Verification items for the finished model (mm, model axes). A direction names the side the tool comes from. Give positions to 0.01 mm unless a question says otherwise; leave off trailing zeros. Write each loop counter-clockwise with the first axis right and the second up, starting at its lowest first coordinate (ties: lowest second). Pieces come first, ordered by that corner, then holes.
from build123d import *

# Parameters (mm, degrees)
SKETCH2_R               = 15.5
SKETCH2_R_2             = 14
BOSS_EXTRUDE1_DEPTH     = 20
SKETCH3_OUTSIDE_W       = 42.638
SKETCH3_OUTSIDE_H       = 42.638
CUT_EXTRUDE1_DEPTH      = 21
SKETCH6_R               = 2
BOSS_EXTRUDE2_DEPTH     = 1.5
CUT_EXTRUDE4_DEPTH      = 21
CUT_EXTRUDE4_DEPTH_BACK = 10
SKETCH9_R               = 2.5
CUT_EXTRUDE5_DEPTH      = 10
FILLET1_R               = 1


with BuildPart() as part:
    # Sketch2 → Boss-Extrude1 (new body)
    with BuildSketch(Plane(origin=(0, 0, 0), x_dir=(1, 0, 0), z_dir=(0, 1, 0))):
        Circle(SKETCH2_R)
        Circle(SKETCH2_R_2, mode=Mode.SUBTRACT)
    boss_extrude1 = extrude(amount=BOSS_EXTRUDE1_DEPTH)

    # Sketch3 outside → Cut-Extrude1 (cut, through all)
    with BuildSketch(Plane(origin=(0, 20, 0), x_dir=(1, 0, 0), z_dir=(0, 1, 0))):
        Rectangle(SKETCH3_OUTSIDE_W, SKETCH3_OUTSIDE_H)
        with BuildLine():
            Line((0, 0), (7.5, 13.564659966))
            ThreePointArc((7.5, 13.564659966), (0, 15.5), (-7.5, 13.564659966))
            Line((-7.5, 13.564659966), (0, 0))
        make_face(mode=Mode.SUBTRACT)
    extrude(amount=-CUT_EXTRUDE1_DEPTH, mode=Mode.SUBTRACT)

    # Sketch6 → Boss-Extrude2 (add, symmetric)
    with BuildSketch(Plane(origin=(0, 7.5, 0), x_dir=(0, 1, 0), z_dir=(-1, 0, 0))):
        with BuildLine():
            Line((-0.5, 20.5), (-0.5, 15.25))
            Line((-0.5, 15.25), (5.5, 15.25))
            Line((5.5, 15.25), (5.5, 20.5))
            ThreePointArc((5.5, 20.5), (2.5, 23.5), (-0.5, 20.5))
        make_face()
        with Locations((2.5, 20.5)):
            Circle(SKETCH6_R, mode=Mode.SUBTRACT)
    boss_extrude2 = extrude(amount=BOSS_EXTRUDE2_DEPTH, both=True)

    # Mirror2: Boss-Extrude1, Boss-Extrude2 across plane
    add(boss_extrude1.mirror(Plane(origin=(0, 0, 0), x_dir=(-0.483870968, 0, 0.875139353), z_dir=(0.875139353, 0, 0.483870968))))
    add(boss_extrude2.mirror(Plane(origin=(0, 0, 0), x_dir=(-0.483870968, 0, 0.875139353), z_dir=(0.875139353, 0, 0.483870968))))

    # Sketch8 → Cut-Extrude4 (cut, two sides)
    with BuildSketch(Plane(origin=(0, 0, 0), x_dir=(1, 0, 0), z_dir=(0, 1, 0))) as cut_extrude4_sk:
        with BuildLine():
            Line((-5.570225317, 14.464528679), (0, 0))
            Line((0, 0), (15.212039463, 2.973862033))
            ThreePointArc((15.212039463, 2.973862033), (-7.5, -13.564659966), (-5.570225317, 14.464528679))
        make_face()
    extrude(amount=CUT_EXTRUDE4_DEPTH, mode=Mode.SUBTRACT)
    extrude(cut_extrude4_sk.sketch, amount=-CUT_EXTRUDE4_DEPTH_BACK, mode=Mode.SUBTRACT)

    # Sketch9 → Cut-Extrude5 (cut)
    with BuildSketch(Plane(origin=(4.354367679, 0, -7.875402257), x_dir=(-0.875139353, 0, -0.483870968), z_dir=(0.483870968, 0, -0.875139353))):
        with Locations((0, 15)):
            Circle(SKETCH9_R)
        with Locations((0, 5)):
            Circle(SKETCH9_R)
    extrude(amount=CUT_EXTRUDE5_DEPTH, mode=Mode.SUBTRACT)

    # Fillet1
    fillet1_edges = [part.edges().sort_by_distance(p)[0] for p in [
        (-1.5, 10, -15.427248621),
        (1.5, 10, -15.427248621),
        (13.863083148, 10, -6.932887251),
        (12.267869828, 10, -9.473614404),
    ]]
    fillet(fillet1_edges, radius=FILLET1_R)


solid = part.part
Item 1: Release check for a two-part mould opening along X. For faces 1 (the face through (15, 13, -9)), 2 (the face through (-5.304, 9.86, -13.774)), 3 (the face through (5.054, 14.042, -13.914)), 4 (the face through (1.75, 9.96, -15.65)) record: released by +X, released by -X, zero draft, split by the parting line, or undercut.
Answer key:
face 1: zero draft
face 2: released by -X
face 3: undercut
face 4: released by +X
Item 2: Sectioned sample at C-C on z = -7. Record the cut outline in (x, y).
Answer key:
outline: (12.12, 0) - (13.83, 0) - (13.83, 7) - (14.25, 7) - (14.25, 13) - (13.83, 13) - (13.83, 20) - (12.12, 20) - close
Item 3: Depth check by flat-ended pin: pin 1 (3 mm diameter, centred on y = 4, z = -8, fed in from -X); pin 2 (12 mm diameter, centred on x = 14, y = 12, fed in from -Z); pin 3 (2 mm diameter, centred on x = 10, y = 8.5, fed in from -Z). Enter the tip coordinate at first touch or a pass-through.
Answer key:
pin 1: stops at x = 10.28
pin 2: stops at z = -13.77
pin 3: stops at z = -12.62
Item 4: Scan lines: line 1 along Y through (x, z) = (0.3, -20.5); line 2 along Z through (x, y) = (0, 10); line 3 along X through (y, z) = (12, -19.25). Record each from-to range of solid material in increasing order.
Answer key:
line 1: y = 7 to 8, 12 to 13
line 2: z = -23.5 to -22.5, -18.5 to -14
line 3: x = -1.5 to 1.5
Item 5: Sectioned sample at A-A on x = 0. Record the cut outline in (y, z).
Answer key:
outline: (0, -15.5) - (7, -15.5) - (7, -20.5) arc R3 ccw to (13, -20.5) - (13, -15.5) - (20, -15.5) - (20, -14) - (0, -14) - close; hole circle Ø4 at (10, -20.5)
Item 6: Sectioned sample at D-D on z = -18. Record the cut outline in (x, y), then the cut area to 3 significant figures.
Answer key:
outline: (-1.5, 7) - (1.5, 7) - (1.5, 13) - (-1.5, 13) - close
area: 18.0 mm2
Item 7: Sectioned sample at B-B on y = 10.75. Record the cut outline in (x, z).
Answer key:
outline: (-5.57, -14.46) arc R15.5 ccw to (-2.35, -15.32) arc R1 cw to (-1.5, -16.31) - (-1.5, -18.65) - (1.5, -18.65) - (1.5, -16.31) arc R1 cw to (2.35, -15.32) arc R15.5 ccw to (11.73, -10.14) arc R1 cw to (13.02, -9.94) - (14.99, -11.19) - (16.59, -8.64) - (14.61, -7.4) arc R1 cw to (14.22, -6.16) arc R15.5 ccw to (15.21, -2.97) - (13.74, -2.69) arc R14 cw to (-5.03, -13.06) - close; (-1.5, -23.4) - (1.5, -23.4) - (1.5, -22.35) - (-1.5, -22.35) - close; (18.13, -13.16) - (19.02, -13.72) - (20.62, -11.17) - (19.73, -10.62) - close
Item 8: Set-up check for faces 5 (the face through (1.5, 10, -18)), 6 (the face through (-1.5, 10, -18)), 7 (the face through (14.7, 10, -11)): record each of +Z, -Z, +X, -X, +Y, -Y from which the full face is reachable in a straight line by a thin tool's end or side.
Answer key:
face 5: -Z, +X, +Y, -Y
face 6: -Z, -X, +Y, -Y
face 7: -Z, +Y, -Y
